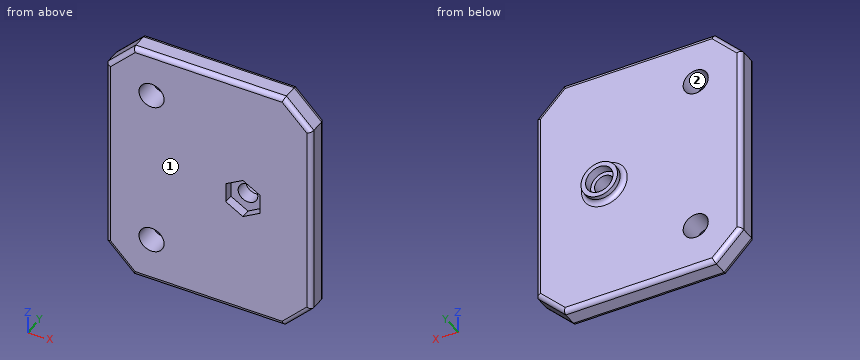
Autodesk Inventor part; units mm, degrees
ref_plane "YZ Plane" through (0, 0, 0) normal (1, 0, 0) x (0, 1, 0)
ref_plane "XZ Plane" through (0, 0, 0) normal (0, 1, 0) x (-1, 0, 0)
ref_plane "XY Plane" through (0, 0, 0) normal (0, 0, 1) x (1, 0, 0)
sketch "スケッチ1" plane through (0, 0, 0) normal (0, 1, 0) x (-1, 0, 0)
  line L0 (22.5, -27.3) -> (-22.5, -27.3)
  line L1 (-22.5, -27.3) -> (-22.5, 27.3)
  line L2 (-22.5, 27.3) -> (22.5, 27.3)
  line L3 (22.5, 27.3) -> (22.5, -27.3)
  line L4 (22.5, -27.3) -> (-22.5, 27.3) construction
  line L5 (-22.5, -27.3) -> (22.5, 27.3) construction
  point P0 (0, 0)
  dimension "d0" = 45
  dimension "d1" = 54.6
extrude "押し出し1" add sketch "スケッチ1" along normal blind 5
sketch "スケッチ2" plane through (0, 5, 0) normal (0, 1, 0) x (1, 0, 0)
  line L0 (-22.5, 27.3) -> (-22.5, -27.3)
  line L1 (-22.5, -27.3) -> (22.5, -27.3)
  line L2 (22.5, 27.3) -> (-22.5, 27.3)
  point P0 (0, 0)
  point P1 (-12.5, -17.3)
  point P2 (-12.5, 17.3)
  dimension "d4" = 10
  dimension "d5" = 10
  dimension "d6" = 10
hole "穴1" at (-12.5, 5, 17.3) at (-12.5, 5, -17.3) direction (0, -1, 0) diameter 5.5 end through all
chamfer "面取り1" distance 6 angle 45 4 edges at (22.5, 2.5, -27.3) (22.5, 2.5, 27.3) (-22.5, 2.5, -27.3) (-22.5, 2.5, 27.3)
sketch "スケッチ5" plane through (0, 5, 0) normal (0, 1, 0) x (1, 0, 0)
  circle A0 centre (-12.5, -17.3) radius 2.75
  point P0 (0, 0)
  point P1 (7.5, 0)
  dimension "d43" = 20
hole "穴2" at (7.5, 5, 0) direction (0, -1, 0) diameter 4.3 end through all
sketch "スケッチ6" plane through (0, 5, 0) normal (0, 1, 0) x (1, 0, 0)
  circle A0 centre (7.5, 0) radius 2.15
  circle A1 centre (7.5, 0) radius 3
  circle A2 centre (7.5, 0) radius 4
  point P0 (0, 0)
  dimension "d51" = 6
  dimension "d52" = 8
extrude "押し出し4" add sketch "スケッチ6" along normal blind 2 contours A2
fillet "フィレット1" radius 1 1 edges at (3.5, 5, 0)
sketch "スケッチ7" plane through (0, 0, 0) normal (0, -1, 0) x (1, 0, 0)
  circle A0 centre (7.5, 0) radius 2.15
  line L0 (7.5, -4.3301) -> (3.75, -2.1651)
  line L1 (3.75, -2.1651) -> (3.75, 2.1651)
  line L2 (3.75, 2.1651) -> (7.5, 4.3301)
  line L3 (7.5, 4.3301) -> (11.25, 2.1651)
  line L4 (11.25, 2.1651) -> (11.25, -2.1651)
  line L5 (11.25, -2.1651) -> (7.5, -4.3301)
  point P0 (0, 0)
  dimension "d56" = 7.5
extrude "押し出し5" cut sketch "スケッチ7" against normal blind 2
fillet "フィレット2" radius 1 16 edges at (-22.5, 5, 0) (-19.5, 5, 24.3) (0, 5, 27.3) (19.5, 5, 24.3) (22.5, 5, 0) (19.5, 5, -24.3) (0, 5, -27.3) (-19.5, 5, -24.3) (0, 0, -27.3) (-19.5, 0, -24.3) (19.5, 0, -24.3) (22.5, 0, 0) (19.5, 0, 24.3) (0, 0, 27.3) (-19.5, 0, 24.3) (-22.5, 0, 0)
properties part number "base1" material "ABS プラスチック"
CAD build for the part. Positions are in the model's coordinates, mm. Face numbers are marked on the shaded views. Round coordinates to 2 decimals unless told otherwise and drop trailing zeros. Write each loop counter-clockwise with the first axis right and the second up, starting at its lowest first coordinate (ties: lowest second). Pieces come first, ordered by that corner, then holes. Notation, with made-up numbers: (-23, -11.5) -> (27, -11.5) arc R24 ccw to (27, 6.5) -> close; hole circle Ø11 at (-25.75, -37.75). An arc over 180 degrees is marked (long way). Answer in a Markdown table with one row per item. Add a question column.
Item 1: Saw through at C-C, the plane z = 17.3. Write the cut outline in (x, y).
Item 2: Saw through at D-D, the plane z = -10. Write the cut outline in (x, y).
Item 3: Saw through at B-B, the plane y = 3. Write the cut outline in (x, z).
Item 4: Saw through at A-A, the plane x = -12.5. Write the cut outline in (y, z), then the cut area to 3 significant figures.
Item 5: Drop flat-ended pins along their axis: pin 1 Ø6.5 at (x, z) = (-12.5, -17.3) entering from +Y; pin 2 Ø4 at (x, z) = (6, 1) entering from -Y. Give the stop position or say it passes through.
Item 6: Drill centre lines: line 1 (Z direction, x = -12.5, y = 1.3); line 2 (X direction, y = 2.3, z = -17.3); line 3 (X direction, y = 3.95, z = 0). Where is each one in solid material? Low to high. Write a range as from..to.
Item 7: Mould opens along Z. For the marked faces 1 and 2 say: pulls with the +Z half, pulls with the -Z half, needs draft (parallel to the pull), parting line crosses it, or undercut.
Findings below:
| question | item | result |
|---|---|---|
| 1 | outline | (-22.5, 1) arc R1 ccw to (-21.5, 0) -> (-15.25, 0) -> (-15.25, 5) -> (-21.5, 5) arc R1 ccw to (-22.5, 4) -> close; (-9.75, 0) -> (21.5, 0) arc R1 ccw to (22.5, 1) -> (22.5, 4) arc R1 ccw to (21.5, 5) -> (-9.75, 5) -> close |
| 2 | outline | (-22.5, 1) arc R1 ccw to (-21.5, 0) -> (21.5, 0) arc R1 ccw to (22.5, 1) -> (22.5, 4) arc R1 ccw to (21.5, 5) -> (-21.5, 5) arc R1 ccw to (-22.5, 4) -> close |
| 3 | outline | (-22.5, -21.3) -> (-16.5, -27.3) -> (16.5, -27.3) -> (22.5, -21.3) -> (22.5, 21.3) -> (16.5, 27.3) -> (-16.5, 27.3) -> (-22.5, 21.3) -> close; hole circle Ø5.5 at (-12.5, -17.3); hole circle Ø5.5 at (-12.5, 17.3); hole circle Ø4.3 at (7.5, 0) |
| 4 | outline | (0, -26.3) arc R1 ccw to (1, -27.3) -> (4, -27.3) arc R1 ccw to (5, -26.3) -> (5, -20.05) -> (0, -20.05) -> close; (0, -14.55) -> (5, -14.55) -> (5, 14.55) -> (0, 14.55) -> close; (0, 20.05) -> (5, 20.05) -> (5, 26.3) arc R1 ccw to (4, 27.3) -> (1, 27.3) arc R1 ccw to (0, 26.3) -> close |
| 4 | area | 217 mm^2 |
| 5 | pin 1 | stops at y = 5 |
| 5 | pin 2 | stops at y = 2 |
| 6 | line 1 | z = -27.3..-20.05, -14.55..14.55, 20.05..27.3 |
| 6 | line 2 | x = -22.5..-15.25, -9.75..22.5 |
| 6 | line 3 | x = -22.5..5.35, 9.65..22.5 |
| 7 | face 1 | needs draft |
| 7 | face 2 | undercut |
